from build123d import *

# Parameters (mm, degrees)
BOSS_EXTRUDE1_DEPTH     = 12.7
CUT_EXTRUDE1_DEPTH      = 110.249530891
CUT_EXTRUDE1_DEPTH_BACK = 110.249530891
SKETCH2_R               = 7.9375


with BuildPart() as part:
    # Sketch1 → Boss-Extrude1 (new, symmetric)
    with BuildSketch(Plane.XY):
        Polygon((-38.1, 0), (38.1, 0), (38.1, 101.6), (25.4, 101.6), (25.4, 50.8), (-25.4, 50.8), (-25.4, 101.6), (-38.1, 101.6), align=None)
    extrude(amount=BOSS_EXTRUDE1_DEPTH, both=True)

    # Sketch2 → Cut-Extrude1 (cut, two sides: drawn at the far end of the back side and taken through both)
    with BuildSketch(Plane(origin=(0, 0, 0), x_dir=(0, 0, -1), z_dir=(1, 0, 0)).offset(-CUT_EXTRUDE1_DEPTH_BACK)):
        with Locations((0, 76.2)):
            Circle(SKETCH2_R)
    extrude(amount=CUT_EXTRUDE1_DEPTH + CUT_EXTRUDE1_DEPTH_BACK, mode=Mode.SUBTRACT)


solid = part.part
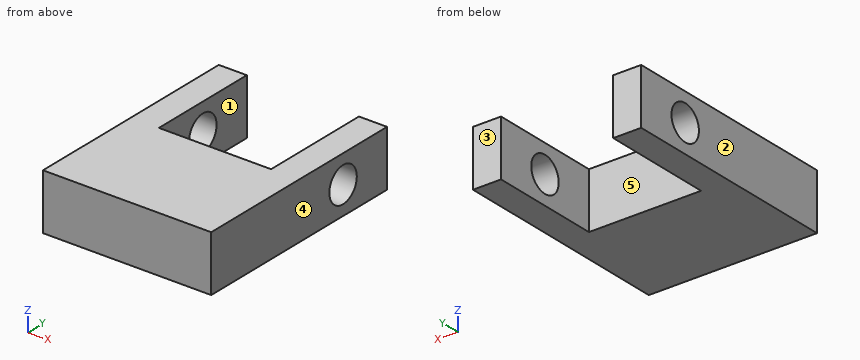
Verification items for the finished model (mm, model axes). Face numbers are marked on the shaded views. A direction names the side the tool comes from. Coordinates: 2 decimals unless noted, no trailing zeros. Loops run counter-clockwise (first coordinate to the right, second up) from the corner with the lowest first, then second, coordinate; pieces in that order, holes last. Notation, with made-up numbers: (74.5, 61.5) -> (110.5, 61.5) arc R13 ccw to (110.5, 80.5) -> close; hole circle Ø5 at (39, 42). An arc over 180 degrees is marked (long way). Write each question's results on one line, items separated by ' | '.
Item 1: Section check A-A, the plane y = 76.2. Enter the section's corners in (x, z).
Found:
outline: (-38.1, -12.7) -> (-25.4, -12.7) -> (-25.4, -7.94) -> (-38.1, -7.94) -> close; (-38.1, 7.94) -> (-25.4, 7.94) -> (-25.4, 12.7) -> (-38.1, 12.7) -> close; (25.4, -12.7) -> (38.1, -12.7) -> (38.1, -7.94) -> (25.4, -7.94) -> close; (25.4, 7.94) -> (38.1, 7.94) -> (38.1, 12.7) -> (25.4, 12.7) -> close
Item 2: Material ranges on L1, parallel to Y at x = -34.75, z = 0; L2, parallel to X at y = 75, z = -10; L3, parallel to Z at x = 32.25, y = 76.2, recorded low to high.
Found:
L1: y = 0 to 68.26, 84.14 to 101.6 | L2: x = -38.1 to -25.4, 25.4 to 38.1 | L3: z = -12.7 to -7.94, 7.94 to 12.7
Item 3: Section check D-D, the plane z = -9. Enter the section's corners in (x, y).
Found:
outline: (-38.1, 0) -> (38.1, 0) -> (38.1, 101.6) -> (25.4, 101.6) -> (25.4, 50.8) -> (-25.4, 50.8) -> (-25.4, 101.6) -> (-38.1, 101.6) -> close
Item 4: Section check B-B, the plane y = 93.5. Enter the section's corners in (x, z).
Found:
outline: (-38.1, -12.7) -> (-25.4, -12.7) -> (-25.4, 12.7) -> (-38.1, 12.7) -> close; (25.4, -12.7) -> (38.1, -12.7) -> (38.1, 12.7) -> (25.4, 12.7) -> close
Item 5: Section check C-C, the plane z = 0. Enter the section's corners in (x, y), plus the area to 3 significant figures.
Found:
outline: (-38.1, 0) -> (38.1, 0) -> (38.1, 68.26) -> (25.4, 68.26) -> (25.4, 50.8) -> (-25.4, 50.8) -> (-25.4, 68.26) -> (-38.1, 68.26) -> close; (-38.1, 84.14) -> (-25.4, 84.14) -> (-25.4, 101.6) -> (-38.1, 101.6) -> close; (25.4, 84.14) -> (38.1, 84.14) -> (38.1, 101.6) -> (25.4, 101.6) -> close | area: 4,760 mm2
Item 6: Tool access check on the marked faces 1 and 2. Record the directions out of +Z, -Z, +X, -X, +Y, -Y that give a thin tool (end or side, any length) a straight path to the whole face; none if there is none.
Found:
face 1: +Z, -Z, +Y | face 2: +Z, -Z, -X, +Y, -Y
Item 7: Gauge pin test, flat end, axial feed: pin 1 (7.5 mm diameter, centred on x = 4.5, z = 3, fed in from +Y). Record the tip position at first contact, or that the pin passes through.
Found:
pin 1: stops at y = 50.8
Item 8: Mould release check, pull along X, two halves, no side actions. Record for the marked faces 3, 4 and 5: +X half, -X half, draft (parallel to the pull), parting line (faces both ways), or undercut.
Found:
face 3: draft | face 4: +X half | face 5: undercut
